Geometry check sheet. Reference: drawing and pictorial views, mm from the part's lowest x, y, z. Round coordinates to 2 decimals unless told otherwise and drop trailing zeros. Order: outer loops, then holes, each group sorted by start corner. A loop starts at its lowest first (then second) coordinate and runs counter-clockwise, first axis right, second up.
(1) Cross-section at B-B on y = 4. Enter the section's corners in (x, z), and give its area (3 significant figures).
(2) Cross-section at A-A on z = 16.75. Enter the section's corners in (x, y) (3 decimals).
(3) Thickness scan on L1, parallel to X at y = 8.5, z = 5.5; L2, parallel to X at y = 11.5, z = 7.5; L3, parallel to Y at x = 17.5, z = 17.5. Record the ranges inside material, lowest first.
(4) Gauge pin test, flat ends, axial feed: P1, Ø6, axis at y = 11, z = 10, coming from the -X side; P2, Ø1.5, axis at y = 5, z = 16, coming from the +X side. Record the tip position at first contact, or that the pin passes through.
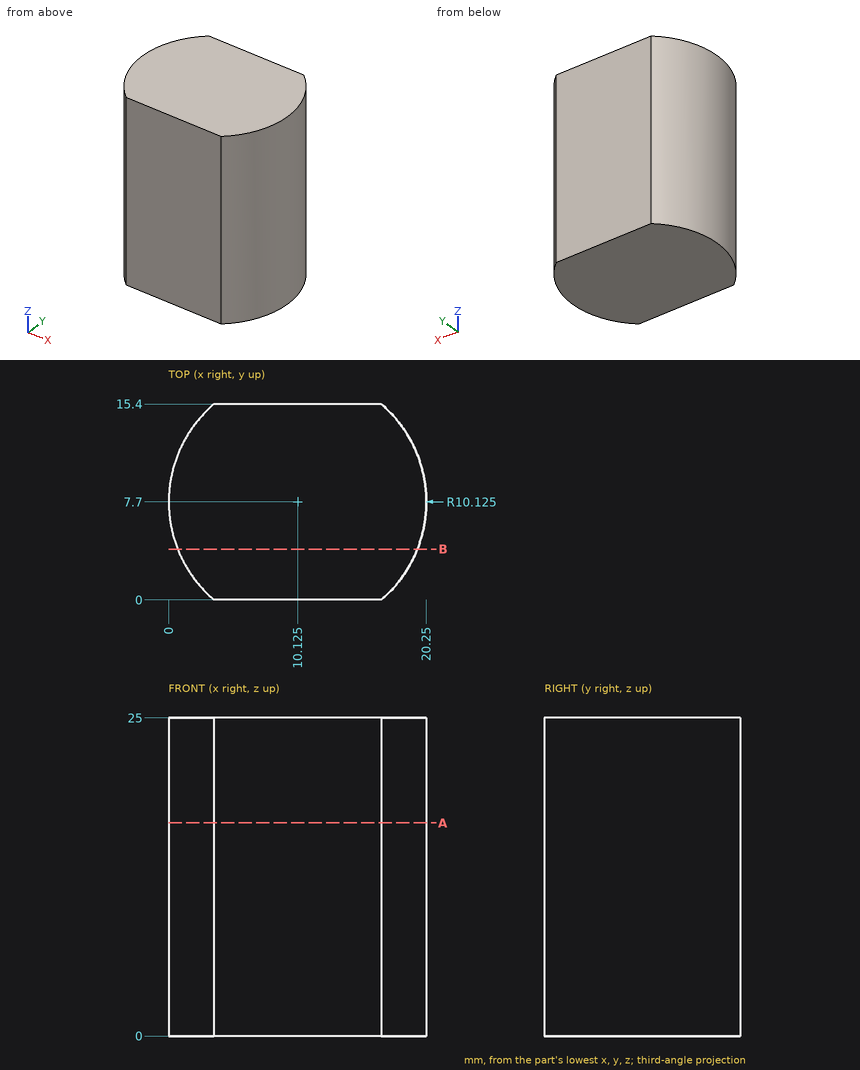
Found:
1. outline: (0.7, 0) - (19.55, 0) - (19.55, 25) - (0.7, 25) - close
1. area: 471 mm2
2. outline: (3.55, 0) - (16.7, 0) arc R10.125 ccw to (16.7, 15.4) - (3.55, 15.4) arc R10.125 ccw to start
3. L1: x = 0.03 to 20.22
3. L2: x = 0.74 to 19.51
3. L3: y = 0.76 to 14.64
4. P1: stops at x = 0
4. P2: stops at x = 20.06
